The listing builds one solid part. Answer for the finished solid, in the listing's coordinates (mm). Round coordinates to 2 decimals unless told otherwise and drop trailing zeros. Write each loop counter-clockwise with the first axis right and the second up, starting at its lowest first coordinate (ties: lowest second). Pieces come first, ordered by that corner, then holes. Notation, with made-up numbers: M 4,87.5 L 20,87.5 A23 cw 20,116.5 Z; hole C 72,-37.75 d9. An arc over 180 degrees is marked long. One line per item, written item: value. Start each with the question number.
(1) Section C-C (y = -7.75) is taken. Determine the outline of the cut face in (x, z).
(2) For a pull along X with two mould halves and no side action, classify faces 1 (the flat face through (-50, -5, 0)), 2 (the cylindrical face through (35, -5, -15)), 3 (the flat face through (-1, -10, 0)) as released by +X, released by -X, zero draft, split by the parting line, or undercut.
(3) Section B-B (x = -40) is taken. Determine the outline of the cut face in (y, z).
(4) Consider probe 1 along Z at (x, y) = (40, -4.5); probe 2 along X at (y, z) = (-9.5, 19); probe 3 along X at (y, z) = (-3.5, 17). Determine where each line is inside the solid, lowest interval first.
(5) Given P1, Ø6, axis at x = 40, z = -15, coming from the +Y side, flat-ended and moving along its own axis, determine where the tip first touches the part or whether it passes through.
(6) Section A-A (z = -15) is taken. Determine the outline of the cut face in (x, y), plus the area to 3 significant figures.
```python
from build123d import *

# Parameters (mm, degrees)
F0_W     = 100
F0_H     = 50
F0_R     = 5
F1_DEPTH = 10
F2_SIZE  = 1
F3_SIZE  = 1
F4_SIZE  = 1


with BuildPart() as f1:
    # F0 (on Front) → F1 (new body)
    with BuildSketch(Plane.XZ):
        Rectangle(F0_W, F0_H)
        with Locations((-40, -15)):
            Circle(F0_R, mode=Mode.SUBTRACT)
        with Locations((40, -15)):
            Circle(F0_R, mode=Mode.SUBTRACT)
        with Locations((-40, 15)):
            Circle(F0_R, mode=Mode.SUBTRACT)
        with Locations((40, 15)):
            Circle(F0_R, mode=Mode.SUBTRACT)
    extrude(amount=F1_DEPTH)

    # F2
    f2_edges = [f1.edges().sort_by_distance(p)[0] for p in [
        (-45, -10, 15),
        (-45, -10, -15),
    ]]
    chamfer(f2_edges, length=F2_SIZE)

    # F3
    f3_edges = [f1.edges().sort_by_distance(p)[0] for p in [
        (35, -10, 15),
        (35, -10, -15),
    ]]
    chamfer(f3_edges, length=F3_SIZE)

    # F4
    f4_edges = [f1.edges().sort_by_distance(p)[0] for p in [
        (35, 0, 15),
        (-45, 0, 15),
        (-45, 0, -15),
        (35, 0, -15),
    ]]
    chamfer(f4_edges, length=F4_SIZE)


solid = f1.part
```
Recorded:
1. outline: M -50,-25 L 50,-25 L 50,25 L -50,25 Z; hole C -40,-15 d10; hole C -40,15 d10; hole C 40,-15 d10; hole C 40,15 d10
2. face 1: released by -X
2. face 2: undercut
2. face 3: zero draft
3. outline: M -10,-25 L 0,-25 L 0,-21 L -1,-20 L -9,-20 L -10,-21 Z; M -10,-9 L -9,-10 L -1,-10 L 0,-9 L 0,9 L -1,10 L -9,10 L -10,9 Z; M -10,21 L -9,20 L -1,20 L 0,21 L 0,25 L -10,25 Z
4. probe 1: z = -25 to -20, -10 to 10, 20 to 25
4. probe 2: x = -50 to -43.77, -36.23 to 36.23, 43.77 to 50
4. probe 3: x = -50 to -44.58, -35.42 to 35.42, 44.58 to 50
5. P1: passes through
6. outline: M -50,-10 L -46,-10 L -45,-9 L -45,-1 L -46,0 L -50,0 Z; M -35,-9 L -34,-10 L 34,-10 L 35,-9 L 35,-1 L 34,0 L -34,0 L -35,-1 Z; M 45,-9 L 46,-10 L 50,-10 L 50,0 L 46,0 L 45,-1 Z
6. area: 796 mm2
